The model under review builds one solid part; all positions refer to its coordinate system, in mm. Face numbers are marked on the shaded views. A direction names the side the tool comes from. Round coordinates to 2 decimals unless told otherwise and drop trailing zeros. Loops run counter-clockwise (first coordinate to the right, second up) from the corner with the lowest first, then second, coordinate; pieces in that order, holes last. Notation, with made-up numbers: M 36,58.5 L 50,58.5 A25 cw 50,79.5 Z; hole C -26.75,13 d6. An arc over 180 degrees is marked long. Use a Markdown table: item, result. Add a question column.
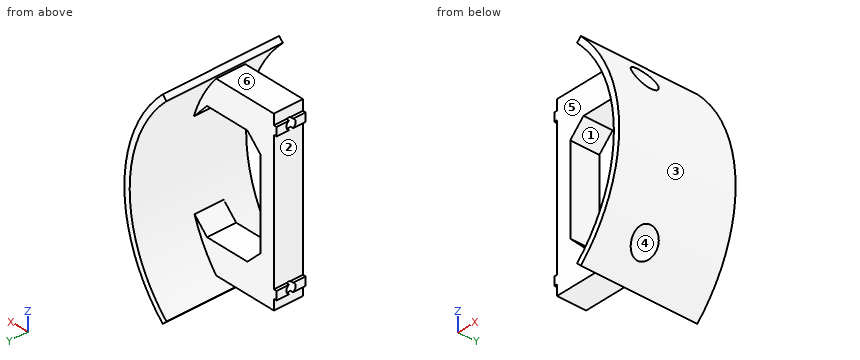
```python
from build123d import *

# Parameters (mm, degrees)
SKETCH1_W           = 2
SKETCH1_H           = 40
MAIN_ANGLE          = 90
SUPPORT_DEPTH       = 10
SKETCH6_W           = 1
SKETCH6_H           = 2.9
FIX_2_DEPTH         = 10
SKETCH9_R           = 1.6
HOLES_DEPTH         = 7
SKETCH10_R          = 4.25
BIGHOLES_DEPTH      = 30.5
BOSS_EXTRUDE3_DEPTH = 10


with BuildPart() as part:
    # Sketch1 → Main (revolve, symmetric)
    with BuildSketch(Plane.XY) as main_sk:
        with Locations((48.5, 20)):
            Rectangle(SKETCH1_W, SKETCH1_H)
    revolve(axis=Axis((0, -0.284703924, 0), (0, 1, 0)), revolution_arc=MAIN_ANGLE / 2)
    revolve(main_sk.sketch, axis=Axis((0, -0.284703924, 0), (0, -1, 0)), revolution_arc=MAIN_ANGLE / 2)

    # Sketch2 → Support (add)
    with BuildSketch(Plane(origin=(0, 10, 0), x_dir=(-1, 0, 0), z_dir=(0, -1, 0))):
        with BuildLine():
            Line((-43.084219849, -20), (-20, -20))
            Line((-20, -20), (-20, 20))
            Line((-20, 20), (-43.084219849, 20))
            ThreePointArc((-43.084219849, 20), (-40.267390497, 25.194984869), (-36.827299657, 30))
            Line((-36.827299657, 30), (-15, 30))
            Line((-15, 30), (-15, -30))
            Line((-15, -30), (-36.827299657, -30))
            ThreePointArc((-36.827299657, -30), (-40.267390497, -25.194984869), (-43.084219849, -20))
        make_face()
    extrude(amount=-SUPPORT_DEPTH)

    # Sketch6 → Fix 2 (add)
    with BuildSketch(Plane(origin=(0, 10, 0), x_dir=(1, 0, 0), z_dir=(0, 1, 0))):
        with Locations((14.5, -25)):
            Rectangle(SKETCH6_W, SKETCH6_H)
        with Locations((14.5, 25)):
            Rectangle(SKETCH6_W, SKETCH6_H)
    extrude(amount=FIX_2_DEPTH)

    # Sketch9 → Holes (cut, through all)
    with BuildSketch(Plane(origin=(20, 0, 0), x_dir=(0, 0, -1), z_dir=(1, 0, 0))):
        with Locations((25, 15)):
            Circle(SKETCH9_R)
        with Locations((-25, 15)):
            Circle(SKETCH9_R)
    extrude(amount=-HOLES_DEPTH, mode=Mode.SUBTRACT)

    # Sketch10 → BigHoles (cut, through all)
    with BuildSketch(Plane(origin=(20, 0, 0), x_dir=(0, 0, -1), z_dir=(1, 0, 0))):
        with Locations((25, 15)):
            Circle(SKETCH10_R)
        with Locations((-25, 15)):
            Circle(SKETCH10_R)
    extrude(amount=BIGHOLES_DEPTH, mode=Mode.SUBTRACT)

    # Sketch11 → Boss-Extrude3 (add)
    with BuildSketch(Plane(origin=(0, 20, 0), x_dir=(1, 0, 0), z_dir=(0, 1, 0))):
        Polygon((20, 20), (25, 20), (20, 15), align=None)
        Polygon((20, -20), (20, -15), (25, -20), align=None)
        Polygon((40.279686395, 20), (45.279686395, 20), (45.279686395, 15), align=None)
        Polygon((40.279686395, -20), (45.279686395, -20), (45.279686395, -14.352700094), align=None)
    extrude(amount=-BOSS_EXTRUDE3_DEPTH)


solid = part.part
```
(1) Consider section B-B, the plane z = -14. Give the boundary of the cut face in (x, y).
(2) Consider section A-A, the plane x = 39. Give the boundary of the cut face in (y, z).
(3) Consider section C-C, the plane x = 16. Give the boundary of the cut face in (y, z), then the cut area to 3 significant figures.
(4) To check wall thickness, follow probe 1 along Z at (x, y) = (29, 15); probe 2 along Y at (x, z) = (17.4, 25); probe 3 along Y at (x, z) = (36, 25). State the ranges of each line that lie inside material, in increasing order.
(5) For the marked faces 1, 2 and 3, list the 3-axis set-ups (+Z, -Z, +X, -X, +Y, -Y) from which the entire face can be reached by the end or side of a thin tool; tool diameter is ignored.
(6) Draft analysis for pull direction Y (two halves, no side actions). For the marked faces 4, 5 and 6, state which applies: released by +Y, released by -Y, zero draft, split by the parting line, or undercut.
(7) Insertion check: pin 1 Ø10 at (x, z) = (34.5, -21) entering from -Y; pin 2 Ø0.8 at (x, y) = (14.5, 11.5) entering from +Z; pin 3 Ø8 at (x, y) = (24.5, 17) entering from +Z; pin 4 Ø1.9 at (y, z) = (15, -25) entering from -X. Each pin has a flat end and moves straight along its axis. Give the tip position at first contact, or say it passes through.
(8) Consider section D-D, the plane y = 24. Give the boundary of the cut face in (x, z).
Found:
| question | item | result |
|---|---|---|
| 1 | outline | M 15,10 L 20,10 L 20,20 L 15,20 Z; M 45.39,0 L 47.48,0 L 47.48,40 L 45.39,40 Z |
| 2 | outline | M 0,-30.48 L 40,-30.48 L 40,-27.12 L 20,-27.12 L 20,-20 L 10,-20 L 10,-27.12 L 0,-27.12 Z; M 0,27.12 L 10,27.12 L 10,20 L 20,20 L 20,27.12 L 40,27.12 L 40,30.48 L 0,30.48 Z; hole C 15,-25 d8.5; hole C 15,25 d8.5 |
| 3 | outline | M 10,-30 L 20,-30 L 20,30 L 10,30 Z; hole C 15,-25 d3.2; hole C 15,25 d3.2 |
| 3 | area | 584 mm^2 |
| 4 | probe 1 | z = -30 to -29.25, -20.75 to -20, 20 to 20.75, 29.25 to 30 |
| 4 | probe 2 | y = 10 to 13.4, 16.6 to 20 |
| 4 | probe 3 | y = 10 to 10.75, 19.25 to 20 |
| 5 | face 1 | +Y, -Y |
| 5 | face 2 | -X, +Y, -Y |
| 5 | face 3 | +X, +Y, -Y |
| 6 | face 4 | undercut |
| 6 | face 5 | released by -Y |
| 6 | face 6 | zero draft |
| 7 | pin 1 | stops at y = 10 |
| 7 | pin 2 | stops at z = 26.45 |
| 7 | pin 3 | stops at z = 30 |
| 7 | pin 4 | passes through |
| 8 | outline | M 33.59,-33.59 L 35,-35 A49.5 ccw 35,35 L 33.59,33.59 A47.5 cw Z |
